Study the drawing (mm; zero at the part's minimum x, y, z) and answer. A direction names the side the tool comes from. Coordinates: 2 decimals unless noted, no trailing zeros. Write each loop counter-clockwise with the first axis right and the second up, starting at its lowest first coordinate (ties: lowest second). Pieces come first, ordered by that corner, then holes. Notation, with made-up numbers: (-30, 65) -> (-19, 65) arc R19 ccw to (-19, 88) -> close; hole circle Ø2 at (-15.75, 39.25). An arc over 180 degrees is marked (long way). Answer in a Markdown table with one row per item. Add a question column.
Item 1: Section A-A on z = 402.5 is taken. Write down the section's boundary in (x, y), then the cut area to 3 significant figures.
Item 2: Given pin 1 Ø4 at (y, z) = (22.5, 288) entering from +X; pin 2 Ø2 at (x, z) = (35, 227) entering from +Y, each flat-ended and moving along its own axis, determine where each tip first touches the part or whether it passes through.
Item 3: Straight lines are drawn through the part: line 1 (X direction, y = 4, z = 12); line 2 (X direction, y = 2, z = 530); line 3 (Z direction, x = 88, y = 5) (1 decimal). For each, find the intervals that lie inside material, in ascending order. Write a range as from..to.
Item 4: Section B-B on y = 16.5 is taken. Write down the section's boundary in (x, z), then the cut area to 3 significant figures.
Item 5: Which of the six approach directions +Z, -Z, +X, -X, +Y, -Y give full straight-line access (tool end or side, diameter ignored) to the marked faces 1 and 2?
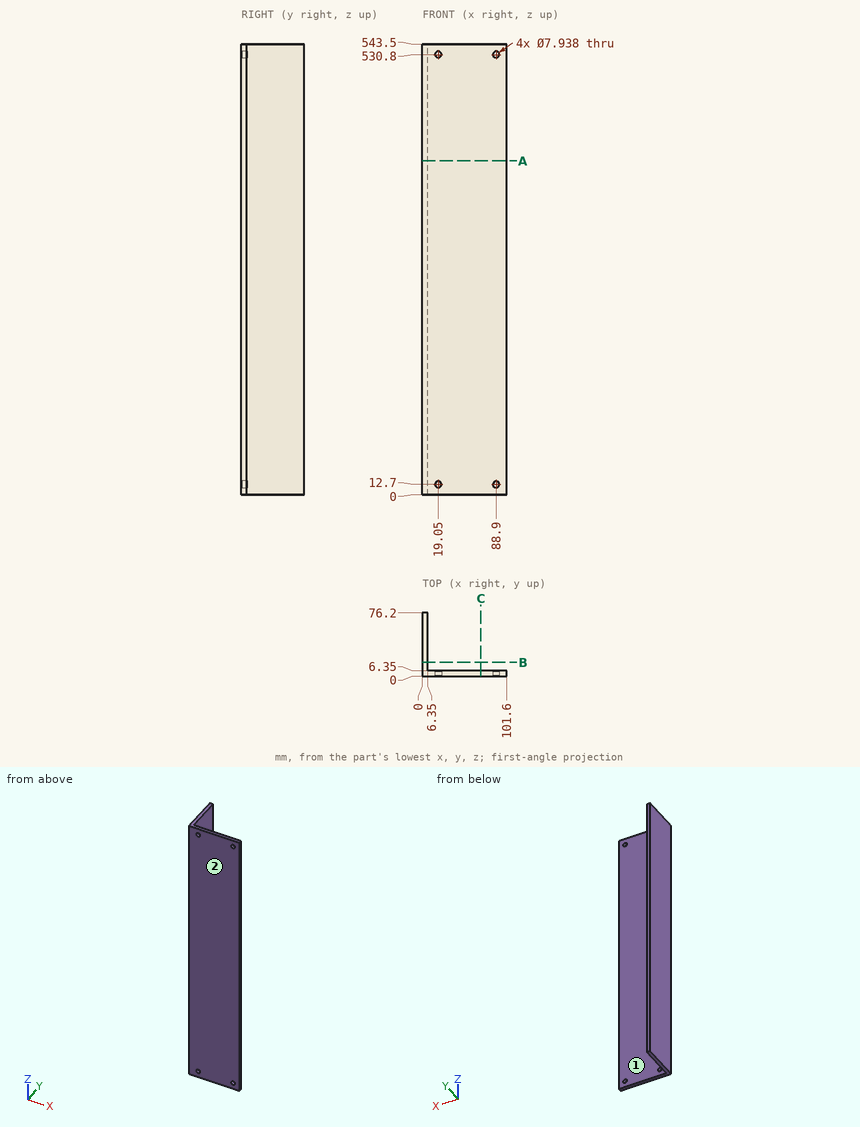
Results below:
| question | item | result |
|---|---|---|
| 1 | outline | (0, 0) -> (101.6, 0) -> (101.6, 6.35) -> (6.35, 6.35) -> (6.35, 76.2) -> (0, 76.2) -> close |
| 1 | area | 1,090 mm2 |
| 2 | pin 1 | stops at x = 6.35 |
| 2 | pin 2 | stops at y = 6.35 |
| 3 | line 1 | x = 0..15.14, 22.96..84.99, 92.81..101.6 |
| 3 | line 2 | x = 0..15.16, 22.94..85.01, 92.79..101.6 |
| 3 | line 3 | z = 0..8.8, 16.6..526.9, 534.7..543.5 |
| 4 | outline | (0, 0) -> (6.35, 0) -> (6.35, 543.5) -> (0, 543.5) -> close |
| 4 | area | 3,450 mm2 |
| 5 | face 1 | +Z, -Z, +X, +Y |
| 5 | face 2 | +Z, -Z, +X, -X, -Y |
